Geometry: final body of the model. Coordinates: model frame, mm. Face numbers are marked on the shaded views. A direction names the side the tool comes from. Give positions to 0.01 mm unless a question says otherwise; leave off trailing zeros. Write each loop counter-clockwise with the first axis right and the second up, starting at its lowest first coordinate (ties: lowest second). Pieces come first, ordered by that corner, then holes. Notation, with made-up numbers: M -24.5,79.25 L 13.5,79.25 A20 cw 13.5,105.25 Z; hole C -27.75,84 d4. An arc over 180 degrees is marked long. One line per question, with ' | ' between items.
from build123d import *

# Parameters (mm, degrees)
F0_R     = 9.235468
F1_DEPTH = 25.4


with BuildPart() as f1:
    # F0 (on Front) → F1 (new body)
    with BuildSketch(Plane.XZ):
        with BuildLine():
            ThreePointArc((1.443592, -28.038119), (20.356194, -19.335083), (28.075257, 0))
            ThreePointArc((28.075257, 0), (21.77593, 17.720861), (5.704746, 27.489561))
            ThreePointArc((5.704746, 27.489561), (-27.992954, 2.148159), (1.443592, -28.038119))
        make_face()
        with BuildLine():
            ThreePointArc((-8.469817, 3.681855), (0, 9.235468), (8.469817, 3.681855))
            Line((8.469817, 3.681855), (17.686794, 3.681855))
            Line((17.686794, 3.681855), (17.686794, -3.681855))
            Line((17.686794, -3.681855), (8.469817, -3.681855))
            ThreePointArc((8.469817, -3.681855), (0, -9.235468), (-8.469817, -3.681855))
            Line((-8.469817, -3.681855), (-17.686794, -3.681855))
            Line((-17.686794, -3.681855), (-17.686794, 3.681855))
            Line((-17.686794, 3.681855), (-8.469817, 3.681855))
        make_face(mode=Mode.SUBTRACT)
        with BuildLine():
            ThreePointArc((5.704746, 27.489561), (21.77593, 17.720861), (28.075257, 0))
            ThreePointArc((28.075257, 0), (20.356194, -19.335083), (1.443592, -28.038119))
            Line((1.443592, -28.038119), (155.082565, -20.127745))
            ThreePointArc((155.082565, -20.127745), (133.891859, -0.022153), (155.038315, 20.129975))
            Line((155.038315, 20.129975), (5.704746, 27.489561))
        make_face()
        with BuildLine():
            ThreePointArc((174.200658, 0), (168.644103, 13.896144), (155.038315, 20.129975))
            ThreePointArc((155.038315, 20.129975), (133.891859, -0.022153), (155.082565, -20.127745))
            ThreePointArc((155.082565, -20.127745), (168.659369, -13.88009), (174.200658, 0))
        make_face()
        with Locations((154.046252, 0)):
            Circle(F0_R, mode=Mode.SUBTRACT)
    extrude(amount=F1_DEPTH)


solid = f1.part
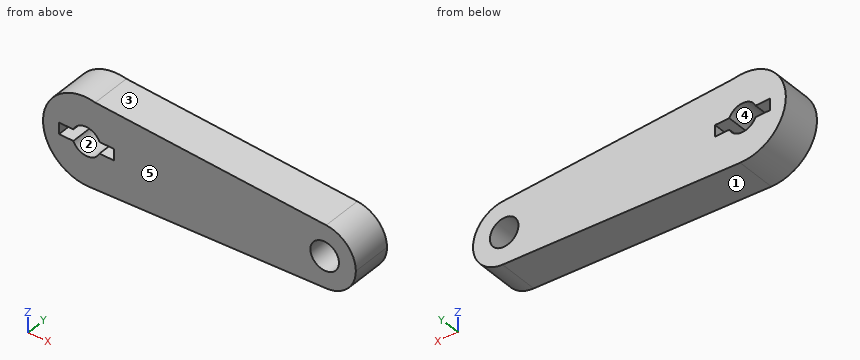
(1) Cut plane C-C, the plane x = 88. Return loops of the section in (y, z).
Working result:
outline: M -25.4,-23.58 L 0,-23.58 L 0,23.43 L -25.4,23.43 Z
(2) Cut plane D-D, the plane z = 23.5. Return loops of the section in (x, y).
Working result:
outline: M -15.36,-25.4 L 86.66,-25.4 L 86.66,0 L -15.36,0 Z
(3) Cut plane B-B, the plane z = -6. Return loops of the section in (x, y), then the cut area to 3 significant figures.
Working result:
outline: M -27.43,-25.4 L -7.02,-25.4 L -7.02,0 L -27.43,0 Z; M 7.02,-25.4 L 147.03,-25.4 L 147.03,0 L 7.02,0 Z; M 161.07,-25.4 L 173.29,-25.4 L 173.29,0 L 161.07,0 Z | area: 4,380 mm^2
(4) Cut plane A-A, the plane y = -17. Return loops of the section in (x, z).
Working result:
outline: M 1.44,-28.04 L 155.08,-20.13 A20.15 ccw 174.2,0 A20.15 ccw 155.04,20.13 L 5.7,27.49 A28.08 ccw long Z; hole M -17.69,-3.68 L -8.47,-3.68 A9.24 ccw 8.47,-3.68 L 17.69,-3.68 L 17.69,3.68 L 8.47,3.68 A9.24 ccw -8.47,3.68 L -17.69,3.68 Z; hole C 154.05,0 d18.47
(5) Draft query along X for the marked faces 3, 4 and 5. Return one class per face: released by +X, released by -X, zero draft, split by the parting line, or undercut.
Working result:
face 3: released by +X | face 4: undercut | face 5: zero draft
(6) Set-up query: the marked faces 1 and 2. Return all of +Z, -Z, +X, -X, +Y, -Y with unobstructed straight access to the full face (end or side cutting, diameter ignored); none if empty.
Working result:
face 1: -Z, +X, +Y, -Y | face 2: +Y, -Y
(7) First-contact query: P1, Ø7.5, axis at x = -12.5, y = -8.5, coming from the +Z side; P2, Ø2, axis at y = -12.5, z = -1.5, coming from the +X side; P3, Ø10, axis at x = 96.5, y = -15, coming from the -Z side. Flat tips, straight axial feed; report the tip coordinate or a pass-through.
Working result:
P1: stops at z = 26.68 | P2: stops at x = 174.19 | P3: stops at z = -23.4
(8) Material intervals for L1, parallel to X at y = -17.75, z = -1; L2, parallel to X at y = -17.5, z = -1.5; L3, parallel to Z at x = 15.5, y = -17, sorted ascending. Write a range as [from, to].
Working result:
L1: x = [-28.06, -17.69], [17.69, 144.87], [163.23, 174.18] | L2: x = [-28.04, -17.69], [17.69, 144.93], [163.16, 174.14] | L3: z = [-27.31, -3.68], [3.68, 27.01]
